Geometry check sheet. Reference: the model listing, model coordinates, mm. Face numbers are marked on the shaded views. Give positions to 0.01 mm unless a question says otherwise; leave off trailing zeros. Order: outer loops, then holes, each group sorted by start corner. A loop starts at its lowest first (then second) coordinate and runs counter-clockwise, first axis right, second up. Notation, with made-up numbers: M -5.5,29.25 L 41.5,29.25 A25 ccw 41.5,68.25 Z; hole C 7,-23.5 d9. An arc over 180 degrees is marked long. Put each result on its own line as item: value. Start each with the question number.
Q1. Section check D-D on x = 65.5. Record the cut outline in (y, z), then the cut area to 3 significant figures.
Q2. Material ranges on L1, parallel to Y at x = 80, z = 9.1; L2, parallel to Y at x = 66.5, z = 1.5; L3, parallel to Y at x = 53, z = 5, recorded low to high.
Q3. Go/stop test with flat-tipped pins: pin 1 (2 mm diameter, centred on y = 110, z = 5, fed in from -X); pin 2 (7 mm diameter, centred on x = 80, y = 10, fed in from -Z); pin 3 (1.5 mm diameter, centred on y = 74.5, z = 4.5, fed in from -X). Record where each tip stops, or that it passes through.
Q4. Section check C-C on y = 70. Record the cut outline in (x, z), then the cut area to 3 significant figures.
Q5. Section check B-B on z = 5. State how many separate pieces and enclosed holes the cut face has, then the cut area to 3 significant figures.
Q6. Mould release check, pull along Y, two halves, no side actions. Record for the marked faces 1, 2 and 3: +Y half, -Y half, draft (parallel to the pull), parting line (faces both ways), or undercut.
Q7. Section check A-A on x = 80. Record the cut outline in (y, z), then the cut area to 3 significant figures.
```python
from build123d import *

# Parameters (mm, degrees)
SKETCH1_R          = 3
EXTRUDE2_DEPTH     = 10
SKETCH5_R          = 5
CUT_EXTRUDE2_DEPTH = 6.5
SKETCH7_R          = 2.25
CUT_EXTRUDE3_DEPTH = 20
SKETCH8_R          = 4
CUT_EXTRUDE4_DEPTH = 10


with BuildPart() as part:
    # Sketch1 → Extrude2 (new body)
    with BuildSketch(Plane.XY):
        with BuildLine():
            ThreePointArc((46.5, 134), (43.916178451, 127.291773917), (37.499940564, 124.050119656))
            Line((37.499940564, 124.050119656), (37.499940564, 100))
            Line((37.499940564, 100), (37.499940564, 91.476734362))
            ThreePointArc((37.499940564, 91.476734362), (58, 70), (37.499940564, 48.523265638))
            Line((37.499940564, 48.523265638), (37.499940564, 39.989097297))
            Line((37.499940564, 39.989097297), (37.499940564, 15.949880344))
            ThreePointArc((37.499940564, 15.949880344), (43.916178451, 12.708226083), (46.5, 6))
            Line((46.5, 6), (46.5, 0))
            Line((46.5, 0), (90, 0))
            Line((90, 0), (90, 140))
            Line((90, 140), (46.5, 140))
            Line((46.5, 140), (46.5, 134))
        make_face()
        with Locations((80, 10)):
            Circle(SKETCH1_R, mode=Mode.SUBTRACT)
        with Locations((66.5, 70)):
            Circle(SKETCH1_R, mode=Mode.SUBTRACT)
        with Locations((80, 130)):
            Circle(SKETCH1_R, mode=Mode.SUBTRACT)
    extrude(amount=EXTRUDE2_DEPTH)

    # Sketch5 → Cut-Extrude2 (cut)
    with BuildSketch(Plane(origin=(0, 0, 0), x_dir=(-1, 0, 0), z_dir=(0, 0, -1))):
        with Locations((-66.5, 70)):
            Circle(SKETCH5_R)
        with Locations((-80, 10)):
            Circle(SKETCH5_R)
        with Locations((-80, 130)):
            Circle(SKETCH5_R)
    extrude(amount=-CUT_EXTRUDE2_DEPTH, mode=Mode.SUBTRACT)

    # Sketch7 → Cut-Extrude3 (cut)
    with BuildSketch(Plane.ZY.offset(-37.499940564)):
        with Locations((5, 110)):
            Circle(SKETCH7_R)
        with Locations((5, 30)):
            Circle(SKETCH7_R)
    extrude(amount=-CUT_EXTRUDE3_DEPTH, mode=Mode.SUBTRACT)

    # Sketch8 → Cut-Extrude4 (cut)
    with BuildSketch(Plane.ZY.offset(-37.499940564)):
        with Locations((5, 41.023265638)):
            Circle(SKETCH8_R)
        with Locations((5, 98.976734362)):
            Circle(SKETCH8_R)
    extrude(amount=-CUT_EXTRUDE4_DEPTH, mode=Mode.SUBTRACT)


solid = part.part
```
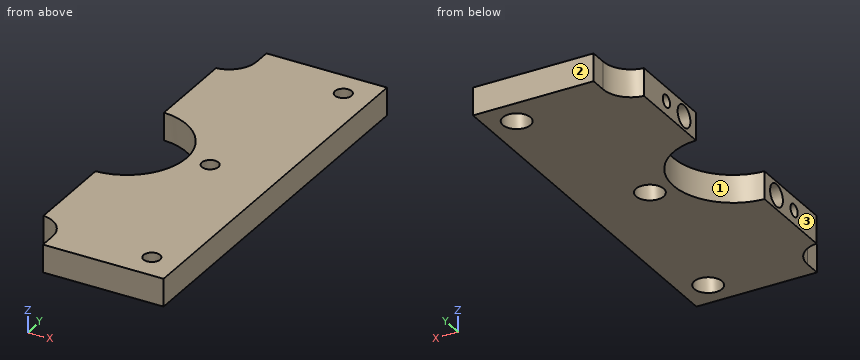
Results found:
1. outline: M 0,0 L 65.1,0 L 65.1,6.5 L 67.17,6.5 L 67.17,10 L 0,10 Z; M 72.83,6.5 L 74.9,6.5 L 74.9,0 L 140,0 L 140,10 L 72.83,10 Z
1. area: 1,320 mm^2
2. L1: y = 0 to 7, 13 to 127, 133 to 140
2. L2: y = 0 to 65, 75 to 140
2. L3: y = 0 to 27.75, 32.25 to 56.22, 83.78 to 107.75, 112.25 to 140
3. pin 1: stops at x = 57.5
3. pin 2: stops at z = 6.5
3. pin 3: stops at x = 57.35
4. outline: M 58,0 L 61.5,0 L 61.5,6.5 L 63.5,6.5 L 63.5,10 L 58,10 Z; M 69.5,6.5 L 71.5,6.5 L 71.5,0 L 90,0 L 90,10 L 69.5,10 Z
4. area: 234 mm^2
5. separate pieces: 1
5. enclosed holes: 3
5. area: 5,850 mm^2
6. face 1: undercut
6. face 2: +Y half
6. face 3: draft
7. outline: M 0,0 L 5,0 L 5,6.5 L 7,6.5 L 7,10 L 0,10 Z; M 13,6.5 L 15,6.5 L 15,0 L 125,0 L 125,6.5 L 127,6.5 L 127,10 L 13,10 Z; M 133,6.5 L 135,6.5 L 135,0 L 140,0 L 140,10 L 133,10 Z
7. area: 1,230 mm^2
